from build123d import *

# Parameters (mm, degrees)
BOSS_EXTRUDE1_DEPTH = 2.2
SKETCH2_R           = 7.5
BOSS_EXTRUDE2_DEPTH = 2.5
SKETCH3_R           = 1.05
CUT_EXTRUDE1_DEPTH  = 15.320963655
CUT_EXTRUDE2_REACH  = 16.321
FILLET1_R           = 1
SKETCH5_R           = 4
BOSS_EXTRUDE3_DEPTH = 3.7
BOSS_EXTRUDE4_DEPTH = 4.1


with BuildPart() as part:
    # Sketch1 → Boss-Extrude1 (new body)
    with BuildSketch(Plane.XY):
        with BuildLine():
            Line((-3.5, 12), (3.5, 12))
            Line((3.5, 12), (3.5, 6.633249581))
            ThreePointArc((3.5, 6.633249581), (7.5, 0), (3.5, -6.633249581))
            Line((3.5, -6.633249581), (3.5, -12))
            Line((3.5, -12), (-3.5, -12))
            Line((-3.5, -12), (-3.5, -6.633249581))
            ThreePointArc((-3.5, -6.633249581), (-7.5, 0), (-3.5, 6.633249581))
            Line((-3.5, 6.633249581), (-3.5, 12))
        make_face()
    extrude(amount=BOSS_EXTRUDE1_DEPTH)

    # Sketch2 → Boss-Extrude2 (add)
    with BuildSketch(Plane.XY.offset(2.2)):
        with Locations(Location((0, 0, 0), (0, 0, 242.181860715))):
            Circle(SKETCH2_R)
    extrude(amount=-BOSS_EXTRUDE2_DEPTH)

    # Sketch3 → Cut-Extrude1 (cut, through all)
    with BuildSketch(Plane(origin=(0, 0, 0), x_dir=(-1, 0, 0), z_dir=(0, 0, -1))):
        with Locations((0, -9.5)):
            Circle(SKETCH3_R)
    extrude(amount=-CUT_EXTRUDE1_DEPTH, mode=Mode.SUBTRACT)

    # Sketch4 → Cut-Extrude2 (cut, up to next)
    with BuildSketch(Plane(origin=(0, 0, 0), x_dir=(-1, 0, 0), z_dir=(0, 0, -1)), mode=Mode.PRIVATE) as cut_extrude2_sk1:
        with BuildLine():
            Line((1.05, 9.745840475), (1.05, 9.245840475))
            ThreePointArc((1.05, 9.245840475), (0, 8.195840475), (-1.05, 9.245840475))
            Line((-1.05, 9.245840475), (-1.05, 9.745840475))
            ThreePointArc((-1.05, 9.745840475), (0, 10.795840475), (1.05, 9.745840475))
        make_face()
    cut_extrude2_tool1 = extrude(cut_extrude2_sk1.sketch, amount=-CUT_EXTRUDE2_REACH, mode=Mode.PRIVATE) & part.part
    add(cut_extrude2_tool1.solids().sort_by_distance((0, 9.49584, 0))[0], mode=Mode.SUBTRACT)

    # Fillet1
    fillet1_edges = [part.edges().sort_by_distance(p)[0] for p in [
        (-3.5, 12, 1.1),
        (3.5, 12, 1.1),
        (3.5, -12, 1.1),
        (-3.5, -12, 1.1),
    ]]
    fillet(fillet1_edges, radius=FILLET1_R)



with BuildPart() as body_2:
    # Sketch5 → Boss-Extrude3 (new body)
    with BuildSketch(Plane.XY.offset(-4.4)):
        Circle(SKETCH5_R)
    extrude(amount=BOSS_EXTRUDE3_DEPTH)


with BuildPart() as part_1:
    add(part.part)

    add(body_2.part)  # Boss-Extrude4 merges body 2
    # Sketch6 → Boss-Extrude4 (add)
    with BuildSketch(Plane.XY.offset(-4.4)):
        with BuildLine():
            Line((-1.295183385, 1.25), (1.295183385, 1.25))
            ThreePointArc((1.295183385, 1.25), (1.8, 0), (1.295183385, -1.25))
            Line((1.295183385, -1.25), (-1.295183385, -1.25))
            ThreePointArc((-1.295183385, -1.25), (-1.8, 0), (-1.295183385, 1.25))
        make_face()
    extrude(amount=BOSS_EXTRUDE4_DEPTH)


solid = part_1.part
Part model, mm, in its own coordinate system. A direction names the side the tool comes from. Coordinates: 2 decimals unless noted, no trailing zeros. Loops run counter-clockwise (first coordinate to the right, second up) from the corner with the lowest first, then second, coordinate; pieces in that order, holes last. Notation, with made-up numbers: M 2,79.5 L 53,79.5 A7 ccw 53,84.5 Z; hole C -4,13.25 d6. An arc over 180 degrees is marked long. Use a Markdown table: item, result. Add a question column.
Q1. Which spindle directions (+Z, -Z, +X, -X, +Y, -Y) get a long thin tool onto all of the face, cutting with end or side? Do faces 1 (the cylindrical face through (3.215, -11.699, 1.115)), 2 (the flat face through (3.5, 9, 1)), 3 (the flat face through (-3.5, -9, 1)), 4 (the flat face through (0, 12, 1)), 5 (the flat face through (0, -2, -0.7)). Say none if no direction does.
Q2. Cut at A-A (x = 0). Write the cut outline in (y, z).
Q3. Mould opens along X. For faces 6 (the cylindrical face through (0.023, 10.796, 1.085)), 7 (the cylindrical face through (-0.023, 8.196, 1.085)), 8 (the flat face through (3.5, -9, 1)), 9 (the flat face through (-3.5, 9, 1)) say: +X half, -X half, draft (parallel to the pull), parting line (faces both ways), or undercut.
Q4. Cut at C-C (y = 0). Write the cut outline in (x, z), and give its area (3 significant figures).
Q5. Pin check, flat tips, straight feed: P1, Ø0.7, axis at y = -8, z = 1.5, coming from the -X side; P2, Ø1.5, axis at x = -2.5, y = 8.5, coming from the -Z side; P3, Ø0.7, axis at y = -9.5, z = 1.5, coming from the +X side. Stop position of each tip, or through.
Q6. Cut at D-D (x = -3.25). Write the cut outline in (y, z), and give its area (3 significant figures).
Q7. Probe L1, parallel to Y at x = 0, z = 1.1; L2, parallel to Z at x = -3.5, y = 0; L3, parallel to Z at x = 4.5, y = 4.5. List the from-to ranges inside material, lowest first.
Q8. Cut at B-B (y = -9.5). Write the cut outline in (x, z).
Worked out:
| question | item | result |
|---|---|---|
| 1 | face 1 | +Z, -Z, +X, -Y |
| 1 | face 2 | +Z, -Z, +X, +Y |
| 1 | face 3 | +Z, -Z, -X, -Y |
| 1 | face 4 | +Z, -Z, +X, -X, +Y |
| 1 | face 5 | none |
| 2 | outline | M -12,0 L -10.55,0 L -10.55,2.2 L -12,2.2 Z; M -8.45,0 L -7.5,0 L -7.5,-0.3 L -1.25,-0.3 L -1.25,-0.7 L -4,-0.7 L -4,-4.4 L 4,-4.4 L 4,-0.7 L 1.25,-0.7 L 1.25,-0.3 L 7.5,-0.3 L 7.5,0 L 8.2,0 L 8.2,2.2 L -8.45,2.2 Z; M 10.8,0 L 12,0 L 12,2.2 L 10.8,2.2 Z |
| 3 | face 6 | undercut |
| 3 | face 7 | undercut |
| 3 | face 8 | +X half |
| 3 | face 9 | -X half |
| 4 | outline | M -7.5,-0.3 L -1.8,-0.3 L -1.8,-0.7 L -4,-0.7 L -4,-4.4 L 4,-4.4 L 4,-0.7 L 1.8,-0.7 L 1.8,-0.3 L 7.5,-0.3 L 7.5,2.2 L -7.5,2.2 Z |
| 4 | area | 68.5 mm2 |
| 5 | P1 | stops at x = -3.5 |
| 5 | P2 | stops at z = 0 |
| 5 | P3 | stops at x = 3.5 |
| 6 | outline | M -11.66,0 L -6.76,0 L -6.76,-0.3 L 6.76,-0.3 L 6.76,0 L 11.66,0 L 11.66,2.2 L -11.66,2.2 Z; M -2.33,-4.4 L 2.33,-4.4 L 2.33,-0.7 L -2.33,-0.7 Z |
| 6 | area | 72.6 mm2 |
| 7 | L1 | y = -12 to -10.55, -8.45 to 8.2, 10.8 to 12 |
| 7 | L2 | z = -4.4 to -0.7, -0.3 to 2.2 |
| 7 | L3 | z = -0.3 to 2.2 |
| 8 | outline | M -3.5,0 L -1.05,0 L -1.05,2.2 L -3.5,2.2 Z; M 1.05,0 L 3.5,0 L 3.5,2.2 L 1.05,2.2 Z |
